Geometry check sheet. Reference: the model listing, model coordinates, mm. A direction names the side the tool comes from. Coordinates: 2 decimals unless noted, no trailing zeros. Loops run counter-clockwise (first coordinate to the right, second up) from the corner with the lowest first, then second, coordinate; pieces in that order, holes last. Notation, with made-up numbers: (78.5, -31.5) - (99.5, -31.5) arc R14 ccw to (99.5, -8.5) - close; hole circle Ø7 at (11, -32). An arc over 180 degrees is marked (long way). Write item = value, one per line. Start each with the question number.
from build123d import *

# Parameters (mm, degrees)
BOSS_EXTRUDE1_DEPTH = 4
SKETCH2_R           = 3.25
SKETCH2_R_2         = 1.5
CUT_EXTRUDE1_DEPTH  = 114.934191532


with BuildPart() as part:
    # Sketch1 → Boss-Extrude1 (new body)
    with BuildSketch(Plane(origin=(0, 0, 0), x_dir=(0, 0, -1), z_dir=(1, 0, 0))):
        Polygon((10, 0), (10, -4), (25, -4), (25, 0), (36, 0), (36, 15), (40, 15), (40, 0), (75, 0), (75, 16), (79, 16), (79, 62), (75, 62), (75, 78), (40, 78), (40, 63), (36, 63), (36, 78), (25, 78), (25, 82), (10, 82), (10, 78), (0, 78), (0, 62), (4, 62), (4, 16), (0, 16), (0, 0), align=None)
    extrude(amount=BOSS_EXTRUDE1_DEPTH)

    # Sketch2 → Cut-Extrude1 (cut, through all)
    with BuildSketch(Plane(origin=(4, 0, 0), x_dir=(0, 0, -1), z_dir=(1, 0, 0))):
        with Locations((65, 10)):
            Circle(SKETCH2_R)
        with Locations((65, 20)):
            Circle(SKETCH2_R_2)
    extrude(amount=-CUT_EXTRUDE1_DEPTH, mode=Mode.SUBTRACT)


solid = part.part
(1) Sectioned sample at C-C on z = -65. Enter the section's corners in (x, y), plus the area to 3 significant figures.
(2) Sectioned sample at D-D on y = 10. Enter the section's corners in (x, z), plus the area to 3 significant figures.
(3) Sectioned sample at A-A on y = 76. Enter the section's corners in (x, z), plus the area to 3 significant figures.
(4) Sectioned sample at B-B on x = 3.2. Count the separate pieces of the cut face and the enclosed holes in it, plus the area to 3 significant figures.
(5) Draft check along Y on faces 6 (the face through (2, 63, -38)), 7 (the face through (4, 40, -39)), 8 (the face through (2, 62, -2)), 9 (the face through (2, 0, -30)). Enter one of: pulls with the +Y half, pulls with the -Y half, needs draft (parallel to the pull), parting line crosses it, or undercut.
(6) Depth check by flat-ended pin: pin 1 (1.2 mm diameter, centred on x = 1, z = -1, fed in from -Y); pin 2 (1.2 mm diameter, centred on x = 2.5, z = -5, fed in from +Y); pin 3 (2 mm diameter, centred on x = 2.5, z = -77.5, fed in from +Y); pin 4 (4 mm diameter, centred on y = 10, z = -65, fed in from +X). Enter the tip coordinate at first touch or a pass-through.
(7) Scan lines: line 1 (Y direction, x = 2.95, z = -65); line 2 (Z direction, x = 2.95, y = 76); line 3 (Y direction, x = 3.5, z = -43). Record each from-to range of solid material in increasing order.
(8) Tool access check on faces 1 (the face through (2, 78, -5)), 2 (the face through (2, -2, -10)), 3 (the face through (2, 0, -57)), 4 (the face through (2, 80, -25)), 5 (the face through (2, 8, -40)). Record the directions out of +Z, -Z, +X, -X, +Y, -Y that give a thin tool (end or side, any length) a straight path to the whole face; none if there is none.
Working result:
q1.outline = (0, 0) - (4, 0) - (4, 6.75) - (0, 6.75) - close; (0, 13.25) - (4, 13.25) - (4, 18.5) - (0, 18.5) - close; (0, 21.5) - (4, 21.5) - (4, 78) - (0, 78) - close
q1.area = 274 mm2
q2.outline = (0, -75) - (4, -75) - (4, -68.25) - (0, -68.25) - close; (0, -61.75) - (4, -61.75) - (4, -40) - (0, -40) - close; (0, -36) - (4, -36) - (4, 0) - (0, 0) - close
q2.area = 258 mm2
q3.outline = (0, -75) - (4, -75) - (4, -40) - (0, -40) - close; (0, -36) - (4, -36) - (4, 0) - (0, 0) - close
q3.area = 284 mm2
q4.separate_pieces = 1
q4.enclosed_holes = 2
q4.area = 5,810 mm2
q5.face_6 = pulls with the +Y half
q5.face_7 = needs draft
q5.face_8 = undercut
q5.face_9 = pulls with the -Y half
q6.pin_1 = 0
q6.pin_2 = 78
q6.pin_3 = 62
q6.pin_4 = through
q7.line_1 = 0 to 6.75, 13.25 to 18.5, 21.5 to 78
q7.line_2 = -75 to -40, -36 to 0
q7.line_3 = 0 to 78
q8.face_1 = +Z, +X, -X, +Y
q8.face_2 = +Z, +X, -X, -Y
q8.face_3 = -Z, +X, -X, -Y
q8.face_4 = -Z, +X, -X, +Y
q8.face_5 = +X, -X, -Y
